For this review, take the finished solid that the model builds, in its own axes (mm). Give positions to 0.01 mm unless a question says otherwise; leave off trailing zeros. Write each loop counter-clockwise with the first axis right and the second up, starting at its lowest first coordinate (ties: lowest second). Pieces come first, ordered by that corner, then holes.
Q1. We need section A-A (y = -0.75). Write out the cut boundary in (x, z).
Q2. Insertion check: P1, Ø1.5, axis at x = -20, z = -14.5, coming from the -Y side; P2, Ø1.5, axis at x = -13.5, y = 0.5, coming from the -Z side; P3, Ø4, axis at x = -23, z = -7.5, coming from the -Y side. Each pin has a flat end and moves straight along its axis. Give the tip position at first contact, or say it passes through.
Q3. For line 1 (X direction, y = 0.25, z = -14); line 2 (X direction, y = 0.7, z = 13.5); line 3 (Z direction, x = 6, y = 2.6), list the stretches that pass through material, from the lowest coordinate up.
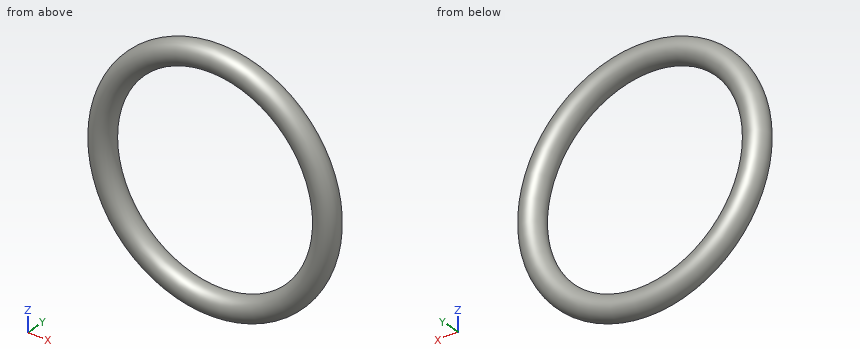
```python
from build123d import *

# Parameters (mm, degrees)
SKE_R = 2.9


with BuildPart() as part:
    # Ske → Revolve 354 (revolve)
    with BuildSketch(Plane.XY, mode=Mode.PRIVATE) as revolve_354_sk:
        with Locations((27.4, 0)):
            Circle(SKE_R)
    revolve(revolve_354_sk.sketch.rotate(Axis((0, 9.409969387, 0), (0, -1, 0)), 180), axis=Axis((0, 9.409969387, 0), (0, -1, 0)))


solid = part.part
```
Computed:
1. outline: circle Ø60.4 at (0, 0); hole circle Ø49.2 at (0, 0)
2. P1: stops at y = -2.15
2. P2: stops at z = -27.46
2. P3: stops at y = -2.64
3. line 1: x = -26.86 to -20.12, 20.12 to 26.86
3. line 2: x = -27.03 to -20.55, 20.55 to 27.03
3. line 3: z = -28.05 to -25.42, 25.42 to 28.05
